For this review, take the finished solid that the model builds, in its own axes (mm). A direction names the side the tool comes from. Round coordinates to 2 decimals unless told otherwise and drop trailing zeros. Order: outer loops, then holes, each group sorted by start corner. A loop starts at its lowest first (then second) coordinate and runs counter-clockwise, first axis right, second up. Notation, with made-up numbers: M 15,-26 L 69,-26 A29 ccw 69,0 Z; hole C -3.5,31.25 d11. An arc over 180 degrees is marked long. Use a Markdown table: item, result.
from build123d import *

# Parameters (mm, degrees)
SKETCH1_W           = 22.5
SKETCH1_H           = 6.975
BOSS_EXTRUDE1_DEPTH = 2.35
SKETCH2_R           = 1.475
BOSS_EXTRUDE2_DEPTH = 8
SKETCH3_W           = 1.5
SKETCH3_H           = 6.975
BOSS_EXTRUDE3_DEPTH = 3.85
SKETCH4_W           = 6.975
SKETCH4_H           = 3
BOSS_EXTRUDE4_DEPTH = 3.5
SKETCH5_W           = 2.1
SKETCH5_H           = 6.975
CUT_EXTRUDE1_DEPTH  = 1.5
SKETCH6_R           = 1.05
BOSS_EXTRUDE5_DEPTH = 6
SKETCH7_R           = 2.4
BOSS_EXTRUDE9_DEPTH = 7.76
FILLET1_R           = 2
FILLET2_R           = 2
FILLET3_R           = 1


with BuildPart() as part:
    # Sketch1 → Boss-Extrude1 (new body)
    with BuildSketch(Plane(origin=(0, 0, 0), x_dir=(1, 0, 0), z_dir=(0, 1, 0))):
        with Locations((-16.71505467, -8.920455339)):
            Rectangle(SKETCH1_W, SKETCH1_H)
    extrude(amount=BOSS_EXTRUDE1_DEPTH)

    # Sketch2 → Boss-Extrude2 (add)
    with BuildSketch(Plane(origin=(0, 2.35, 0), x_dir=(1, 0, 0), z_dir=(0, 1, 0))):
        with Locations(Location((-25.31505467, -10.457955339, 0), (0, 0, 270))):
            Circle(SKETCH2_R)
        with Locations(Location((-8.11505467, -10.457955339, 0), (0, 0, 270))):
            Circle(SKETCH2_R)
    extrude(amount=BOSS_EXTRUDE2_DEPTH)

    # Sketch3 → Boss-Extrude3 (add)
    with BuildSketch(Plane(origin=(0, 0, 0), x_dir=(-1, 0, 0), z_dir=(0, -1, 0))):
        with Locations((6.21505467, -8.920455339)):
            Rectangle(SKETCH3_W, SKETCH3_H)
    extrude(amount=BOSS_EXTRUDE3_DEPTH)

    # Sketch4 → Boss-Extrude4 (add)
    with BuildSketch(Plane(origin=(-5.46505467, 0, 0), x_dir=(0, 0, -1), z_dir=(1, 0, 0))):
        with Locations((-8.920455339, -2.35)):
            Rectangle(SKETCH4_W, SKETCH4_H)
    extrude(amount=BOSS_EXTRUDE4_DEPTH)

    # Sketch5 → Cut-Extrude1 (cut)
    with BuildSketch(Plane(origin=(0, -0.85, 0), x_dir=(1, 0, 0), z_dir=(0, 1, 0))):
        with Locations((-4.41505467, -8.920455339)):
            Rectangle(SKETCH5_W, SKETCH5_H)
    extrude(amount=-CUT_EXTRUDE1_DEPTH, mode=Mode.SUBTRACT)

    # Sketch6 → Boss-Extrude5 (add)
    with BuildSketch(Plane(origin=(0, 2.35, 0), x_dir=(1, 0, 0), z_dir=(0, 1, 0))):
        with Locations(Location((-7.76505467, -7.007955339, 0), (0, 0, 270))):
            Circle(SKETCH6_R)
        with Locations(Location((-25.66505467, -7.007955339, 0), (0, 0, 270))):
            Circle(SKETCH6_R)
    extrude(amount=BOSS_EXTRUDE5_DEPTH)

    # Sketch7 → Boss-Extrude9 (add)
    with BuildSketch(Plane(origin=(0, 0, 0), x_dir=(-1, 0, 0), z_dir=(0, -1, 0))):
        with Locations(Location((16.71505467, -9.097955339, 0), (0, 0, 270))):
            Circle(SKETCH7_R)
        with Locations(Location((24.68505467, -9.097955339, 0), (0, 0, 270))):
            Circle(SKETCH7_R)
    extrude(amount=BOSS_EXTRUDE9_DEPTH)

    # Fillet1
    fillet1_edges = [part.edges().sort_by_distance(p)[0] for p in [
        (-6.96505467, -3.85, 8.920455339),
    ]]
    fillet(fillet1_edges, radius=FILLET1_R)

    # Fillet2
    fillet2_edges = [part.edges().sort_by_distance(p)[0] for p in [
        (-1.96505467, -3.85, 8.920455339),
    ]]
    fillet(fillet2_edges, radius=FILLET2_R)

    # Fillet3
    fillet3_edges = [part.edges().sort_by_distance(p)[0] for p in [
        (-1.96505467, -0.85, 8.920455339),
    ]]
    fillet(fillet3_edges, radius=FILLET3_R - 0.0001)  # a hair under: the kernel refuses the full size


solid = part.part
Q1. Add section B-B (x = -14). Write out the cut boundary in (y, z), then the cut area to 3 significant figures.
Determined:
| item | result |
|---|---|
| outline | M 0,5.43 L 2.35,5.43 L 2.35,12.41 L 0,12.41 Z |
| area | 16.4 mm^2 |
Q2. Machinability: for faces 1 (the flat face through (-4, -2.35, 9)), 2 (the cylindrical face through (-6.364, -3.28, 8.872)), 3 (the flat face through (-26, 8.35, 7)), which of the approach directions +Z, -Z, +X, -X, +Y, -Y give a long, thin tool a straight path to every point of the face, cutting with its end or side? Answer none if there is none.
Determined:
| item | result |
|---|---|
| face 1 | +Z, -Z, +Y |
| face 2 | +Z, -Z, -Y |
| face 3 | -Z, +X, -X, +Y |
Q3. Add section D-D (y = -4.75). Write out the cut boundary in (x, z).
Determined:
| item | result |
|---|---|
| outline | C -24.69,9.1 d4.8; C -16.72,9.1 d4.8 |
Q4. Draft analysis for pull direction Z (two halves, no side actions). For faces 4 (the flat face through (-15, 1, 12.408)), 5 (the flat face through (-8, 8.35, 7)), 6 (the cylindrical face through (-9.555, 6.294, 10.138)), 7 (the cylindrical face through (-26.69, 5.31, 6.78)), state which applies: pulls with the +Z half, pulls with the -Z half, needs draft (parallel to the pull), parting line crosses it, or undercut.
Determined:
| item | result |
|---|---|
| face 4 | pulls with the +Z half |
| face 5 | needs draft |
| face 6 | undercut |
| face 7 | undercut |
Q5. Wall thickness on line 1 along X through (y, z) = (-0.75, 9.25); line 2 along X through (y, z) = (9.25, 10.5); line 3 along X through (y, z) = (7.5, 7): over which ranges is each line inside the solid? List them lowest first. Write a range as [from, to].
Determined:
| item | result |
|---|---|
| line 1 | x = [-27.08, -22.29], [-19.11, -14.32], [-6.97, -5.47] |
| line 2 | x = [-26.79, -23.84], [-9.59, -6.64] |
| line 3 | x = [-26.72, -24.62], [-8.82, -6.72] |
Q6. Add section C-C (y = 1). Write out the cut boundary in (x, z).
Determined:
| item | result |
|---|---|
| outline | M -27.97,5.43 L -5.47,5.43 L -5.47,12.41 L -27.97,12.41 Z |
Q7. Clearance check with flat-ended pins moving along their axes: pin 1 (0.8 mm diameter, centred on y = -1.5, z = 8.5, fed in from -X); pin 2 (4 mm diameter, centred on y = 3.5, z = 9, fed in from +X); pin 3 (3 mm diameter, centred on x = -23, y = 5, fed in from -Z); pin 4 (5 mm diameter, centred on x = -19, y = 8, fed in from +Z). State where each tip first meets the part, or that it passes through.
Determined:
| item | result |
|---|---|
| pin 1 | stops at x = -27.08 |
| pin 2 | stops at x = -5.47 |
| pin 3 | stops at z = 9.23 |
| pin 4 | passes through |
